```python
from build123d import *

# Parameters (mm, degrees)
SKETCH10_R          = 3
BOSS_EXTRUDE2_DEPTH = 3.5


with BuildPart() as part:
    # Sketch1 → Revolve1 (revolve)
    with BuildSketch(Plane.XY, mode=Mode.PRIVATE) as revolve1_sk:
        Polygon((0, 0), (5, 0), (1, 5.45), (0, 5.45), align=None)
    revolve(revolve1_sk.sketch.rotate(Axis((0, -3.7, 0), (0, 1, 0)), 90), axis=Axis((0, -3.7, 0), (0, 1, 0)))

    # Sketch3 → Cut-Revolve1 (revolve, cut)
    with BuildSketch(Plane.XY, mode=Mode.PRIVATE) as cut_revolve1_sk:
        Polygon((-1.65, 3.4), (-1.65, 2.4), (-3, 0), (0, 0), (0, 3.4), align=None)
        Polygon((-0.25, 5.45), (0, 5.45), (0, 3.4), (-1.65, 3.4), align=None)
    revolve(cut_revolve1_sk.sketch.rotate(Axis((0, 0, 0), (0, 1, 0)), 270), axis=Axis((0, 0, 0), (0, 1, 0)), mode=Mode.SUBTRACT)

    # Sketch10 → Boss-Extrude2 (add)
    with BuildSketch(Plane.XZ):
        Polygon((5.731649919, -0.693918255), (3.466775796, 4.616795308), (-2.264874122, 5.310713562), (-5.731649919, 0.693918255), (-3.466775796, -4.616795308), (2.264874122, -5.310713562), align=None)
        with Locations(Location((0, 0, 0), (0, 0, 270))):
            Circle(SKETCH10_R, mode=Mode.SUBTRACT)
    extrude(amount=BOSS_EXTRUDE2_DEPTH)


solid = part.part
```
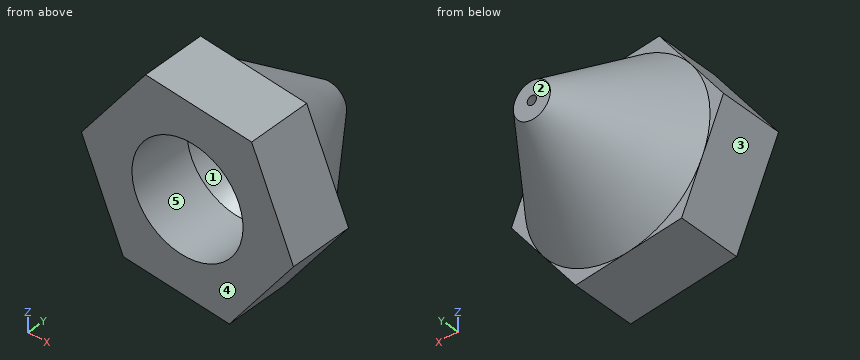
Check sheet for the modelled part. Datum: model origin and axes. Units: mm. Face numbers are marked on the shaded views. A direction names the side the tool comes from. Coordinates: 2 decimals unless noted, no trailing zeros. Write each loop counter-clockwise with the first axis right and the second up, starting at its lowest first coordinate (ties: lowest second). Pieces come first, ordered by that corner, then holes. Notation, with made-up numbers: (52.5, -5.5) - (97.5, -5.5) arc R13 cw to (97.5, 19.5) - close; hole circle Ø6 at (64, 50.25). An arc over 180 degrees is marked (long way). One line per question, with ' | ' between items.
Item 1: Gauge pin test, flat ends, axial feed: P1, Ø4, axis at y = 2.5, z = -2, coming from the +X side; P2, Ø1.5, axis at x = 0.5, y = 0.5, coming from the +Z side; P3, Ø6, axis at x = -3, z = 4, coming from the +Y side. Record the tip position at first contact, or that the pin passes through.
Determined:
P1: stops at x = 4.35 | P2: stops at z = 5.04 | P3: stops at y = 4.09
Item 2: Sectioned sample at C-C on z = 0. Record the boundary of the cut face in (x, y).
Determined:
outline: (-5.44, -3.5) - (-3, -3.5) - (-3, 0) - (-1.65, 2.4) - (-1.65, 3.4) - (-0.25, 5.45) - (-1, 5.45) - (-5, 0) - (-5.44, 0) - close; (0.25, 5.45) - (1.65, 3.4) - (1.65, 2.4) - (3, 0) - (3, -3.5) - (5.44, -3.5) - (5.44, 0) - (5, 0) - (1, 5.45) - close
Item 3: Mould release check, pull along Z, two halves, no side actions. Record for the marked faces 1, 2 and 3: pulls with the +Z half, pulls with the -Z half, needs draft (parallel to the pull), parting line crosses it, or undercut.
Determined:
face 1: undercut | face 2: needs draft | face 3: pulls with the -Z half
Item 4: Access from +Z, -Z, +X, -X, +Y, -Y to the whole of each face (thin tool, end or side, straight path). Record for the marked faces 4 and 5.
Determined:
face 4: +Z, -Z, +X, -X, -Y | face 5: -Y
Item 5: Sectioned sample at D-D on y = 4.25. Record the boundary of the cut face in (x, z), plus the area to 3 significant figures.
Determined:
outline: circle Ø3.76 at (0, 0); hole circle Ø2.14 at (0, 0) | area: 7.52 mm2
Item 6: Thickness scan on line 1 (X direction, y = -2.45, z = 0); line 2 (Z direction, x = 0, y = -1.9); line 3 (X direction, y = 2.75, z = 0.25). Record the ranges inside material, lowest first. Write a range as [from, to].
Determined:
line 1: x = [-5.44, -3], [3, 5.44] | line 2: z = [-5.04, -3], [3, 5.04] | line 3: x = [-2.97, -1.63], [1.63, 2.97]
Item 7: Sectioned sample at A-A on y = -3. Record the boundary of the cut face in (x, z).
Determined:
outline: (-5.73, 0.69) - (-3.47, -4.62) - (2.26, -5.31) - (5.73, -0.69) - (3.47, 4.62) - (-2.26, 5.31) - close; hole circle Ø6 at (0, 0)
